Work out the finished part from the listing and answer in its coordinate system (mm). Face numbers are marked on the shaded views. A direction names the side the tool comes from. Coordinates: 2 decimals unless noted, no trailing zeros. Order: outer loops, then holes, each group sorted by start corner. A loop starts at its lowest first (then second) coordinate and runs counter-clockwise, first axis right, second up. Notation, with made-up numbers: (16, 32.5) - (51, 32.5) arc R21 ccw to (51, 55.5) - close; hole circle Ø1 at (55, 83.25). An arc over 180 degrees is marked (long way). Answer as a JSON object with one key per item and string values. Group by question number.
1) Section A-A (y = 0) is taken. Give the vertices of the cut face in (x, z), plus the area to 3 significant figures.
2) A tool of negligible diameter and unlimited length cuts with its end or side. For the marked faces 4, 5 and 6, from which of +Z, -Z, +X, -X, +Y, -Y can it reach the whole face along a straight path? Write none if from no direction.
3) Each of these flat-tipped pins is pushed along its axis until it touches: P1, Ø6, axis at x = -90, z = 5.5, coming from the -Y side; P2, Ø2, axis at x = -94, y = 4.5, coming from the +Z side; P3, Ø4, axis at x = -52.5, z = -16, coming from the -Y side; P4, Ø5, axis at y = -14, z = -21, coming from the +X side. Where does it stop, or does it pass through?
4) Section C-C (z = 54) is taken. Give the vertices of the cut face in (x, y), plus the area to 3 significant figures.
5) Find the intervals of material crossed by line 1 along X through (y, z) = (9.5, 52); line 2 along Y through (x, z) = (-64.25, -50.8); line 3 along Z through (x, y) = (-67, -50), in increasing order.
6) Section D-D (x = -38) is taken. Give the vertices of the cut face in (y, z).
7) The mould has two halves that part along Z. Classify the marked faces 1, 2 and 3: released by +Z, released by -Z, zero draft, split by the parting line, or undercut.
Autodesk Inventor part; units mm, degrees
ref_plane "YZ Plane" through (0, 0, 0) normal (1, 0, 0) x (0, 1, 0)
ref_plane "XZ Plane" through (0, 0, 0) normal (0, 1, 0) x (-1, 0, 0)
ref_plane "XY Plane" through (0, 0, 0) normal (0, 0, 1) x (1, 0, 0)
sketch "Sketch1" plane through (0, 0, 0) normal (0, 0, 1) x (1, 0, 0)
  line L0 (0, 0) -> (0, 31.5)
  line L1 (0, 31.5) -> (-60, 31.5)
  line L2 (-60, 31.5) -> (-60, 62)
  line L3 (-60, 62) -> (-72, 62)
  line L4 (-72, 62) -> (-72, 31.5)
  line L5 (-72, 31.5) -> (-122, 31.5)
  line L6 (-122, 31.5) -> (-122, 25.5)
  line L7 (-122, 25.5) -> (-147, 25.5)
  line L8 (-147, 25.5) -> (-147, 0)
  line L9 (-147, 0) -> (0, 0)
  dimension "d0" = 31.5
  dimension "d1" = 60
  dimension "d2" = 30.5
  dimension "d3" = 12
  dimension "d4" = 30.5
  dimension "d5" = 50
  dimension "d6" = 6
  dimension "d7" = 25
revolve "Revolution1" add sketch "Sketch1" angle 360 about axis through (-147, 0, 0) along (1, 0, 0)
sketch "Sketch2" plane through (-60, 0, 0) normal (1, 0, 0) x (0, 0, -1)
  circle A0 centre (0, 50.8) radius 6.35
  circle A1 centre (-50.8, 0) radius 6.35
  circle A2 centre (50.8, 0) radius 6.35
  circle A3 centre (0, -50.8) radius 6.35
  line L0 (0, 0) -> (0, 50.8) construction
  line L1 (0, 0) -> (0, 50.8) construction
  line L2 (0, 0) -> (50.8, 0) construction
  line L3 (0, 0) -> (0, -50.8) construction
  line L4 (0, 0) -> (-50.8, 0) construction
  dimension "d9" = 12.7
  dimension "d10" = 50.8
  dimension "d11" = 12.7
  dimension "d12" = 12.7
  dimension "d13" = 12.7
extrude "Extrusion1" cut sketch "Sketch2" against normal through all
sketch "Sketch3" plane through (0, 0, 0) normal (1, 0, 0) x (0, 0, -1)
  circle A0 centre (0, 0) radius 16
  dimension "d16" = 32
extrude "Extrusion2" cut sketch "Sketch3" against normal blind 60
properties part number "pilot"
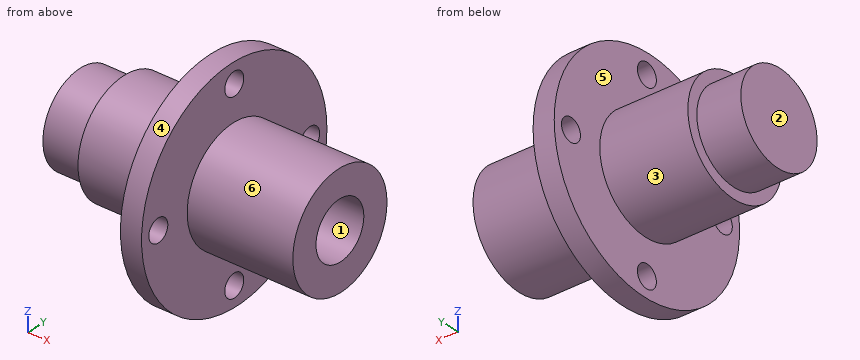
Report:
{
 "1": {"outline": "(-147, -25.5) - (-122, -25.5) - (-122, -31.5) - (-72, -31.5) - (-72, -44.45) - (-60, -44.45) - (-60, -31.5) - (0, -31.5) - (0, -16) - (-60, -16) - (-60, 16) - (0, 16) - (0, 31.5) - (-60, 31.5) - (-60, 44.45) - (-72, 44.45) - (-72, 31.5) - (-122, 31.5) - (-122, 25.5) - (-147, 25.5) - close; (-72, -62) - (-60, -62) - (-60, -57.15) - (-72, -57.15) - close; (-72, 57.15) - (-60, 57.15) - (-60, 62) - (-72, 62) - close", "area": "7,470 mm²"},
 "2": {"face 4": "+X, -X", "face 5": "-X", "face 6": "+X"},
 "3": {"P1": "stops at y = -31.4", "P2": "stops at z = 31.3", "P3": "stops at y = -28.22", "P4": "stops at x = 0"},
 "4": {"outline": "(-72, -30.46) - (-60, -30.46) - (-60, -5.48) - (-72, -5.48) - close; (-72, 5.48) - (-60, 5.48) - (-60, 30.46) - (-72, 30.46) - close", "area": "599 mm²"},
 "5": {"line 1": "x = -72 to -60", "line 2": "y = -35.54 to -6.35, 6.35 to 35.54", "line 3": "z = -36.66 to -6.3, 6.3 to 36.66"},
 "6": {"outline": "circle Ø63 at (0, 0); hole circle Ø32 at (0, 0)"},
 "7": {"face 1": "undercut", "face 2": "zero draft", "face 3": "split by the parting line"}
}
